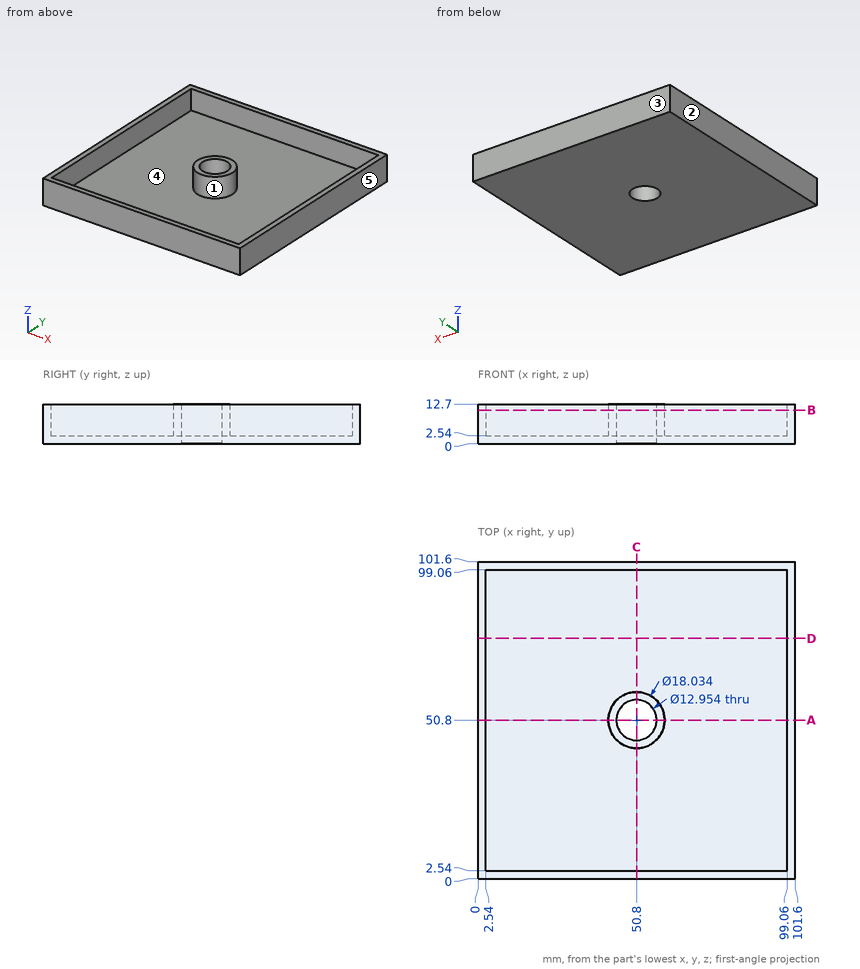
Input: dimensioned drawing with shaded views. Units: mm. Origin: part minimum x, y, z. A direction names the side the tool comes from. Give positions to 0.01 mm unless a question says otherwise; leave off trailing zeros. Write each loop counter-clockwise with the first axis right and the second up, starting at its lowest first coordinate (ties: lowest second). Pieces come first, ordered by that corner, then holes. Notation, with made-up numbers: M 40.5,67.25 L 84.5,67.25 A16 cw 84.5,82.25 Z; hole C 37,2 d6. An arc over 180 degrees is marked long. Write item = value, one per line. Start each with the question number.
1) Cut plane B-B on z = 10.75. Return the cut outline in (x, y), then the cut area to 3 significant figures.
2) Cut plane D-D on y = 77. Return the cut outline in (x, z), then the cut area to 3 significant figures.
3) Reachability of the marked faces 1 and 2 from +Z, -Z, +X, -X, +Y, -Y: full face, straight path, thin tool, end or side. Return the list, or none.
4) Draft query along Y for the marked faces 3, 4 and 5. Return one class per face: +Y half, -Y half, draft (parallel to the pull), parting line (faces both ways), or undercut.
5) Cut plane A-A on y = 50.8. Return the cut outline in (x, z).
6) First-contact query: pin 1 Ø4 at (x, y) = (13.5, 88) entering from -Z; pin 2 Ø2 at (x, y) = (31.5, 60.5) entering from +Z. Flat tips, straight axial feed; report the tip coordinate or a pass-through.
7) Material intervals for line 1 along Y through (x, z) = (50.8, 8.75); line 2 along Y through (x, z) = (16, 11.5), sorted ascending. Write a range as [from, to].
Solved:
q1.outline = M 0,0 L 101.6,0 L 101.6,101.6 L 0,101.6 Z; C 50.8,50.8 d18.03; hole M 2.54,2.54 L 99.06,2.54 L 99.06,99.06 L 2.54,99.06 Z; hole C 50.8,50.8 d12.95
q1.area = 1,130 mm2
q2.outline = M 0,0 L 101.6,0 L 101.6,12.7 L 99.06,12.7 L 99.06,2.54 L 2.54,2.54 L 2.54,12.7 L 0,12.7 Z
q2.area = 310 mm2
q3.face_1 = +Z
q3.face_2 = +Z, -Z, -X, +Y, -Y
q4.face_3 = +Y half
q4.face_4 = undercut
q4.face_5 = draft
q5.outline = M 0,0 L 44.32,0 L 44.32,12.7 L 41.78,12.7 L 41.78,2.54 L 2.54,2.54 L 2.54,12.7 L 0,12.7 Z; M 57.28,0 L 101.6,0 L 101.6,12.7 L 99.06,12.7 L 99.06,2.54 L 59.82,2.54 L 59.82,12.7 L 57.28,12.7 Z
q6.pin_1 = 0
q6.pin_2 = 2.54
q7.line_1 = [0, 2.54], [41.78, 44.32], [57.28, 59.82], [99.06, 101.6]
q7.line_2 = [0, 2.54], [99.06, 101.6]
